Autodesk Inventor part; units mm, degrees
ref_plane "YZ Plane" through (0, 0, 0) normal (1, 0, 0) x (0, 1, 0)
ref_plane "XZ Plane" through (0, 0, 0) normal (0, 1, 0) x (-1, 0, 0)
ref_plane "XY Plane" through (0, 0, 0) normal (0, 0, 1) x (1, 0, 0)
sketch "Sketch1" plane through (0, 0, 0) normal (0, 1, 0) x (-1, 0, 0)
  line L0 (0, 0) -> (0, -320.8) construction
  line L1 (0, -320.8) -> (47.15, -320.8) construction
  line L2 (0, -170.8) -> (10.5, -170.8) construction
  line L3 (0, -20.8) -> (9.5, -20.8) construction
  line L4 (0, -15.3) -> (12.6, -15.3) construction
  line L5 (0, 0) -> (10.5, 0) construction
  line L6 (10.5, 0) -> (10.5, -15.3)
  line L7 (12.6, -15.3) -> (9.5, -20.8)
  line L8 (12.6, -15.3) -> (10.5, -15.3)
  line L9 (10.5, -170.8) -> (9.5, -20.8)
  arc A0 (10.5, -170.8) -> (47.15, -320.8) centre (344.907, -168.5706) ccw
  line L10 (7.8613, 0) -> (9, -170.8)
  arc A1 (9, -170.8) -> (45.4663, -320.8) centre (344.907, -168.5706) ccw
  line L11 (10.5, 0) -> (7.8613, 0)
  arc A2 (45.4663, -320.8) -> (47.15, -320.8) centre (46.3082, -320.372) ccw
  dimension "d0" = 47.15
  dimension "d1" = 10.5
  dimension "d2" = 9.5
  dimension "d3" = 12.6
  dimension "d4" = 10.5
  dimension "d5" = 150
  dimension "d6" = 150
  dimension "d7" = 5.5
  dimension "d8" = 15.3
  dimension "d9" = 1.5
revolve "Revolution1" add sketch "Sketch1" angle 360 about axis through (0, 0, 0) along (0, 0, -1)
thread "Thread1"
equation "\"d0\" = Flare_Diameter"
equation "\"d1\" = Transition_Diameter"
equation "\"d2\" = Tail_Diameter"
equation "\"d3\" = Mount_Flange_Diameter"
equation "\"d4\" = Mount_Diameter"
equation "\"d5\" = Flare_Length"
equation "\"d6\" = Transition_Length"
equation "\"d7\" = Mount_Flange_Length"
equation "\"d8\" = Mount_Length"
equation "\"d9\" = Bell_Thickness"
equation "\"Bell_Thickness\" = 1.5"
equation "\"Flare_Length\" = 150"
equation "\"Transition_Length\" = 150"
equation "\"Transition_Diameter\" = 10.5"
equation "\"Flare_Diameter\" = 47.15"
equation "\"Mount_Length\" = 15.3"
equation "\"Mount_Diameter\" = 10.5"
equation "\"Mount_Flange_Length\" = 5.5"
equation "\"Mount_Flange_Diameter\" = 12.6"
equation "\"Tail_Diameter\" = 9.5"
properties part number "Horn_A" material "Steel, Cast"
Input: part model. Units: mm. Frame: model coordinates. A direction names the side the tool comes from. Give positions to 0.01 mm unless a question says otherwise; leave off trailing zeros. Loops run counter-clockwise (first coordinate to the right, second up) from the corner with the lowest first, then second, coordinate; pieces in that order, holes last. Notation, with made-up numbers: M 46,62 L 63,62 A13 ccw 63,83 Z; hole C 57,-37 d1. An arc over 180 degrees is marked long. Use one line per item in the form item = value.
1. Line query: L1, parallel to X at y = 0.5, z = -12.5; L2, parallel to X at y = 0, z = -302.5; L3, parallel to Y at x = 6.5, z = -24. Output: solid intervals per line, ascending.
Numbers:
L1 = -10.49 to -7.93, 7.93 to 10.49
L2 = -38.48 to -36.85, 36.85 to 38.48
L3 = -6.96 to -4.7, 4.7 to 6.96
2. First-contact query: pin 1 (12 mm diameter, centred on x = -13, y = 12, fed in from +Z); pin 2 (3 mm diameter, centred on y = -6.5, z = -102, fed in from -X); pin 3 (10 mm diameter, centred on x = 3.5, z = -222.5, fed in from +Y). Flat tips, straight axial feed; report the tip coordinate or a pass-through.
Numbers:
pin_1 = -15.3
pin_2 = -8.71
pin_3 = 15.58
3. Pull-direction query (X, two-part tool) for faces 1 (the face through (-10, 3.2, -7.8)), 2 (the face through (-8.05, 2.53, -86.6)), 3 (the face through (2.9, 10.3, -15.3)); classes: released by +X, released by -X, zero draft, split by the parting line, or undercut.
Numbers:
face_1 = split by the parting line
face_2 = undercut
face_3 = zero draft
4. Section query A-A, the plane z = -138. Return the cut outline in (x, y).
Numbers:
outline = C 0,0 d20.56; hole C 0,0 d17.56
5. Reachability of faces 4 (the face through (1, 8, 0)), 5 (the face through (2.17, -9.77, -96.85)) from +Z, -Z, +X, -X, +Y, -Y: full face, straight path, thin tool, end or side. Return the list, or none.
Numbers:
face_4 = +Z, +X, -X, +Y, -Y
face_5 = none
6. Section query B-B, the plane z = -24. Return the cut outline in (x, y).
Numbers:
outline = C 0,0 d19.04; hole C 0,0 d16.04
